Work out the finished part from the listing and answer in its coordinate system (mm). Round coordinates to 2 decimals unless told otherwise and drop trailing zeros. Order: outer loops, then holes, each group sorted by start corner. A loop starts at its lowest first (then second) coordinate and runs counter-clockwise, first axis right, second up. Notation, with made-up numbers: M 10.25,2 L 39.25,2 A26 cw 39.25,32 Z; hole C 53,63.5 d9. An arc over 180 degrees is marked long. Answer as a JSON object with one key per item and string values. Group by question number.
from build123d import *

# Parameters (mm, degrees)
SKETCH1_W                 = 215
SKETCH1_H                 = 250
BOSS_EXTRUDE1_DEPTH       = 3.175
SKETCH2_R                 = 25.4
CUT_EXTRUDE1_DEPTH        = 165.897940027
SKETCH3_W                 = 11
SKETCH3_H                 = 25
CUT_EXTRUDE2_DEPTH        = 165.897940027
FILLET1_R                 = 2
SKETCH4_W                 = 20
SKETCH4_H                 = 6
CUT_EXTRUDE3_DEPTH        = 165.897940027
LPATTERN1_COUNT           = 2
LPATTERN1_PITCH           = 160
LPATTERN1_COPY_1_SKETCH_W = 20
LPATTERN1_COPY_1_SKETCH_H = 6
LPATTERN1_COPY_1_DEPTH    = 165.897940027
M3X0_5_TAPPED_HOLE1_D     = 2.5
SKETCH9_W                 = 6
SKETCH9_H                 = 25
CUT_EXTRUDE4_DEPTH        = 165.897940027


with BuildPart() as part:
    # Sketch1 → Boss-Extrude1 (new body)
    with BuildSketch(Plane.XY):
        Rectangle(SKETCH1_W, SKETCH1_H)
    extrude(amount=BOSS_EXTRUDE1_DEPTH)

    # Sketch2 → Cut-Extrude1 (cut, through all)
    with BuildSketch(Plane.XY.offset(3.175)):
        with Locations((0, 135)):
            Circle(SKETCH2_R)
    extrude(amount=-CUT_EXTRUDE1_DEPTH, mode=Mode.SUBTRACT)

    # Sketch3 → Cut-Extrude2 (cut, through all)
    with BuildSketch(Plane.XY.offset(3.175)):
        with Locations((-102, 112.5)):
            Rectangle(SKETCH3_W, SKETCH3_H)
    cut_extrude2 = extrude(amount=-CUT_EXTRUDE2_DEPTH, mode=Mode.SUBTRACT)

    # Mirror1: Cut-Extrude2 across plane
    add(cut_extrude2.mirror(Plane(origin=(0, 0, 0), x_dir=(0, 0, 1), z_dir=(1, 0, 0))), mode=Mode.SUBTRACT)

    # Fillet1
    fillet1_edges = [part.edges().sort_by_distance(p)[0] for p in [
        (23.348661632, 125, 1.5875),
        (-23.348661632, 125, 1.5875),
        (-107.5, 100, 1.5875),
        (-96.5, 125, 1.5875),
        (-96.5, 100, 1.5875),
        (107.5, 100, 1.5875),
        (96.5, 100, 1.5875),
        (96.5, 125, 1.5875),
        (107.5, -125, 1.5875),
        (-107.5, -125, 1.5875),
    ]]
    fillet(fillet1_edges, radius=FILLET1_R)

    # Sketch4 → Cut-Extrude3 (cut, through all)
    with BuildSketch(Plane(origin=(0, 0, 0), x_dir=(-1, 0, 0), z_dir=(0, 0, -1))):
        with Locations((-60, -40.5)):
            Rectangle(SKETCH4_W, SKETCH4_H)
        with Locations((-60, -62.375)):
            Rectangle(SKETCH4_W, SKETCH4_H)
    cut_extrude3 = extrude(amount=-CUT_EXTRUDE3_DEPTH, mode=Mode.SUBTRACT)

    # Mirror2: Cut-Extrude3 across plane
    add(cut_extrude3.mirror(Plane(origin=(0, 0, 0), x_dir=(0, 0, 1), z_dir=(1, 0, 0))), mode=Mode.SUBTRACT)

    # LPattern1: Cut-Extrude3 ×2
    with Locations(*[(0, i * LPATTERN1_PITCH, 0) for i in range(1, LPATTERN1_COUNT)]):
        add(cut_extrude3, mode=Mode.SUBTRACT)

    # LPattern1 copy 1 sketch → LPattern1 copy 1 (cut, through all)
    with BuildSketch(Plane(origin=(0, 160, 0), x_dir=(1, 0, 0), z_dir=(0, 0, -1))):
        with Locations((-60, 40.5)):
            Rectangle(LPATTERN1_COPY_1_SKETCH_W, LPATTERN1_COPY_1_SKETCH_H)
        with Locations((-60, 62.375)):
            Rectangle(LPATTERN1_COPY_1_SKETCH_W, LPATTERN1_COPY_1_SKETCH_H)
    extrude(amount=-LPATTERN1_COPY_1_DEPTH, mode=Mode.SUBTRACT)

    # M3x0.5 Tapped Hole1 (through all)
    with Locations(Plane(origin=(0, 0, 0), x_dir=(-1, 0, 0), z_dir=(0, 0, -1))):
        with Locations((-104.5, 87), (104.5, 87), (104.5, -122), (-104.5, -122)):
            Hole(M3X0_5_TAPPED_HOLE1_D / 2)

    # Sketch9 → Cut-Extrude4 (cut, through all)
    with BuildSketch(Plane(origin=(0, 0, 0), x_dir=(-1, 0, 0), z_dir=(0, 0, -1))):
        with Locations((75.5, 37.5)):
            Rectangle(SKETCH9_W, SKETCH9_H)
        with Locations((99.5, 37.5)):
            Rectangle(SKETCH9_W, SKETCH9_H)
    cut_extrude4 = extrude(amount=-CUT_EXTRUDE4_DEPTH, mode=Mode.SUBTRACT)

    # Mirror3: Cut-Extrude4 across plane
    add(cut_extrude4.mirror(Plane(origin=(0, 0, 0), x_dir=(0, 0, 1), z_dir=(1, 0, 0))), mode=Mode.SUBTRACT)


solid = part.part
Item 1: Find section C-C (z = 1.85). Give the number of separate pieces and of enclosed holes in the cut face, and give its area (3 significant figures).
Item 2: Find section B-B (x = 62). Give the vertices of the cut face in (y, z) (3 decimals), and give its area (3 significant figures).
Item 3: Each of these flat-tipped pins is pushed along its axis until it touches: pin 1 (1.6 mm diameter, centred on y = 119, z = 1, fed in from +X); pin 2 (1 mm diameter, centred on x = -2, z = 2, fed in from +Y); pin 3 (4 mm diameter, centred on x = -104.5, y = -122, fed in from +Z) (3 decimals). Where does it stop, or does it pass through?
Item 4: Consider L1, parallel to X at y = -122, z = 0.85; L2, parallel to Y at x = 66, z = 0.5 (3 decimals); L3, parallel to Y at x = 104.5, z = 1.55. Determine where each line is inside the solid, lowest interval first.
Item 5: The mould has two halves that part along X. Classify faces 1 (the flat face through (-2, 2, 0)), 2 (the cylindrical face through (-0.397, 109.603, 1.61)): +X half, -X half, draft (parallel to the pull), parting line (faces both ways), or undercut.
Item 6: Find section D-D (x = -4.5). Give the vertices of the cut face in (y, z) (3 decimals).
Item 7: Find section A-A (y = 31.5). Give the vertices of the cut face in (x, z) (3 decimals), and give its area (3 significant figures).
Responses:
{
 "1": {"separate pieces": "1", "enclosed holes": "16", "area": "51,100 mm^2"},
 "2": {"outline": "M -125,0 L -65.375,0 L -65.375,3.175 L -125,3.175 Z; M -59.375,0 L -43.5,0 L -43.5,3.175 L -59.375,3.175 Z; M -37.5,0 L 94.625,0 L 94.625,3.175 L -37.5,3.175 Z; M 100.625,0 L 116.5,0 L 116.5,3.175 L 100.625,3.175 Z; M 122.5,0 L 125,0 L 125,3.175 L 122.5,3.175 Z", "area": "718 mm^2"},
 "3": {"pin 1": "stops at x = 96.5", "pin 2": "stops at y = 109.72", "pin 3": "stops at z = 3.175"},
 "4": {"L1": "x = -107.5 to -105.75, -103.25 to 103.25, 105.75 to 107.5", "L2": "y = -125 to -65.375, -59.375 to -43.5, -37.5 to 94.625, 100.625 to 116.5, 122.5 to 125", "L3": "y = -125 to -123.25, -120.75 to 85.75, 88.25 to 100"},
 "5": {"face 1": "draft", "face 2": "undercut"},
 "6": {"outline": "M -125,0 L 110.002,0 L 110.002,3.175 L -125,3.175 Z"},
 "7": {"outline": "M -107.5,0 L -102.5,0 L -102.5,3.175 L -107.5,3.175 Z; M -96.5,0 L -78.5,0 L -78.5,3.175 L -96.5,3.175 Z; M -72.5,0 L 72.5,0 L 72.5,3.175 L -72.5,3.175 Z; M 78.5,0 L 96.5,0 L 96.5,3.175 L 78.5,3.175 Z; M 102.5,0 L 107.5,0 L 107.5,3.175 L 102.5,3.175 Z", "area": "606 mm^2"}
}
